from build123d import *

# Parameters (mm, degrees)
SKETCH1_W           = 25
SKETCH1_H           = 25
BOSS_EXTRUDE1_DEPTH = 1
SKETCH2_W           = 21
SKETCH2_H           = 5
BOSS_EXTRUDE2_DEPTH = 2
SKETCH3_W           = 8
SKETCH3_H           = 8
BOSS_EXTRUDE3_DEPTH = 2
SKETCH5_R           = 3.5
BOSS_EXTRUDE4_DEPTH = 1
BOSS_EXTRUDE5_DEPTH = 1
SKETCH7_R           = 1
CUT_EXTRUDE1_DEPTH  = 1


with BuildPart() as part:
    # Sketch1 → Boss-Extrude1 (new body)
    with BuildSketch(Plane(origin=(0, 0, 0), x_dir=(0, 0, -1), z_dir=(1, 0, 0))):
        with Locations((12.5, 12.5)):
            Rectangle(SKETCH1_W, SKETCH1_H)
    extrude(amount=BOSS_EXTRUDE1_DEPTH)

    # Sketch2 → Boss-Extrude2 (add)
    with BuildSketch(Plane(origin=(1, 0, 0), x_dir=(0, 0, -1), z_dir=(1, 0, 0))):
        with Locations((12.5, 3.5)):
            Rectangle(SKETCH2_W, SKETCH2_H)
    extrude(amount=BOSS_EXTRUDE2_DEPTH)

    # Sketch3 → Boss-Extrude3 (add)
    with BuildSketch(Plane.ZY):
        with Locations((-12.5, 10)):
            Rectangle(SKETCH3_W, SKETCH3_H)
    extrude(amount=BOSS_EXTRUDE3_DEPTH)

    # Sketch5 → Boss-Extrude4 (add)
    with BuildSketch(Plane.ZY.offset(2)):
        with Locations((-12.5, 10)):
            Circle(SKETCH5_R)
    extrude(amount=BOSS_EXTRUDE4_DEPTH)

    # Sketch6 → Boss-Extrude5 (add)
    with BuildSketch(Plane.ZY):
        Polygon((-16, 23.363866642), (-9, 23.363866642), (-9, 19.363866642), (-10, 19.363866642), (-10, 14), (-15, 14), (-15, 19.363866642), (-16, 19.363866642), align=None)
    extrude(amount=BOSS_EXTRUDE5_DEPTH)

    # Sketch7 → Cut-Extrude1 (cut)
    with BuildSketch(Plane.ZY):
        with Locations((-23.5, 23.5)):
            Circle(SKETCH7_R)
        with Locations((-1.5, 23.5)):
            Circle(SKETCH7_R)
        with Locations((-1.5, 9.5)):
            Circle(SKETCH7_R)
        with Locations((-23.5, 9.5)):
            Circle(SKETCH7_R)
    extrude(amount=-CUT_EXTRUDE1_DEPTH, mode=Mode.SUBTRACT)


solid = part.part
CAD build for the part. Positions are in the model's coordinates, mm. A direction names the side the tool comes from. Round coordinates to 2 decimals unless told otherwise and drop trailing zeros. Write each loop counter-clockwise with the first axis right and the second up, starting at its lowest first coordinate (ties: lowest second). Pieces come first, ordered by that corner, then holes.
(1) 3-axis set-ups, long thin cutter, end or side, ignore diameter. For faces 1 (the face through (2, 1, -12)), 2 (the face through (2, 3, -23)), 3 (the face through (-1.2, 14, -12.6)), 4 (the face through (-0.5, 16.6, -15)): which of +Z, -Z, +X, -X, +Y, -Y reach the whole face in a straight line?
(2) Drop flat-ended pins along their axis: P1, Ø1.2, axis at y = 23.5, z = -1.5, coming from the -X side; P2, Ø12.5, axis at y = 17, z = -16.5, coming from the +X side; P3, Ø3, axis at y = 19.5, z = -4, coming from the -X side; P4, Ø1.6, axis at x = -1, y = 11, coming from the -Z side. Give the stop position or say it passes through.
(3) Slice it at C-C, the plane z = -19.25. Write the cut outline in (x, y).
(4) Mould opens along Y. For faces 5 (the face through (2, 6, -12)), 6 (the face through (-0.5, 19.364, -9.5)), 7 (the face through (3, 4, -12)) say: pulls with the +Y half, pulls with the -Y half, needs draft (parallel to the pull), parting line crosses it, or undercut.
(5) Slice it at B-B, the plane y = 9.5. Write the cut outline in (x, z), and give its area (3 significant figures).
(6) Slice it at A-A, the plane z = -1.5. Write the cut outline in (x, y).
(7) Slice it at D-D, the plane x = 2.5. Write the cut outline in (y, z).
(8) Probe line 1 along Y through (x, z) = (0.3, -23.5); line 2 along Y through (x, z) = (2.5, -22); line 3 along X through (y, z) = (13.5, -3). List the from-to ranges inside material, lowest first.
From the geometry:
1. face 1: +Z, -Z, +X, -Y
1. face 2: -Z, +X, +Y, -Y
1. face 3: -X
1. face 4: -Z, -X
2. P1: passes through
2. P2: stops at x = 1
2. P3: stops at x = 0
2. P4: stops at z = -16.5
3. outline: (0, 0) - (1, 0) - (1, 1) - (3, 1) - (3, 6) - (1, 6) - (1, 25) - (0, 25) - close
4. face 5: pulls with the +Y half
4. face 6: undercut
4. face 7: needs draft
5. outline: (-3, -15.96) - (-2, -15.96) - (-2, -16.5) - (0, -16.5) - (0, -22.5) - (1, -22.5) - (1, -2.5) - (0, -2.5) - (0, -8.5) - (-2, -8.5) - (-2, -9.04) - (-3, -9.04) - close; (0, -25) - (1, -25) - (1, -24.5) - (0, -24.5) - close; (0, -0.5) - (1, -0.5) - (1, 0) - (0, 0) - close
5. area: 43.9 mm2
6. outline: (0, 0) - (1, 0) - (1, 8.5) - (0, 8.5) - close; (0, 10.5) - (1, 10.5) - (1, 22.5) - (0, 22.5) - close; (0, 24.5) - (1, 24.5) - (1, 25) - (0, 25) - close
7. outline: (1, -23) - (6, -23) - (6, -2) - (1, -2) - close
8. line 1: y = 0 to 8.5, 10.5 to 22.5, 24.5 to 25
8. line 2: y = 1 to 6
8. line 3: x = 0 to 1
